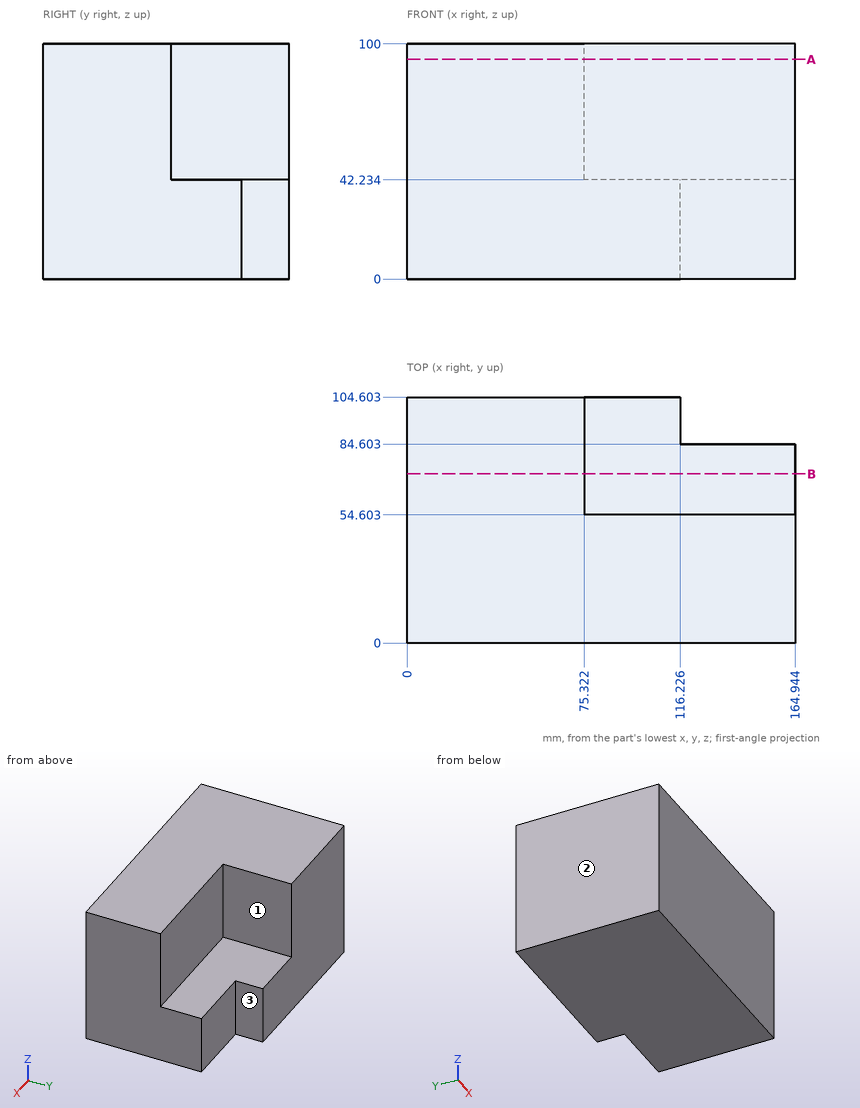
Geometry check sheet. Reference: drawing and pictorial views, mm from the part's lowest x, y, z. A direction names the side the tool comes from. Coordinates: 2 decimals unless noted, no trailing zeros. Order: outer loops, then holes, each group sorted by start corner. A loop starts at its lowest first (then second) coordinate and runs counter-clockwise, first axis right, second up. Notation, with made-up numbers: M 71,49.25 L 109,49.25 A16 cw 109,74.25 Z; hole C 60.25,-37.75 d3. An arc over 180 degrees is marked long. Return JSON: item names as keys, results as strings.
1) Thickness scan on L1, parallel to Z at x = 108, y = 68; L2, parallel to X at y = 94, z = 36; L3, parallel to Y at x = 147, z = 42.5. Record the ranges inside material, lowest first. Write a range as [from, to].
Answer list:
{"L1": "[0, 42.23]", "L2": "[0, 116.23]", "L3": "[0, 54.6]"}
2) Access from +Z, -Z, +X, -X, +Y, -Y to the whole of each face (thin tool, end or side, straight path). Record for the marked faces 1, 2 and 3.
Answer list:
{"face 1": "+Z, +X, +Y", "face 2": "+Z, -Z, -X, +Y, -Y", "face 3": "+Z, -Z, +X, +Y"}
3) Cross-section at A-A, the plane z = 93.5. Record the boundary of the cut face in (x, y), and give its area (3 significant figures).
Answer list:
{"outline": "M 0,0 L 164.94,0 L 164.94,54.6 L 75.32,54.6 L 75.32,104.6 L 0,104.6 Z", "area": "12,800 mm2"}
4) Cross-section at B-B, the plane y = 72. Record the boundary of the cut face in (x, z), and give its area (3 significant figures).
Answer list:
{"outline": "M 0,0 L 164.94,0 L 164.94,42.23 L 75.32,42.23 L 75.32,100 L 0,100 Z", "area": "11,300 mm2"}
5) Gauge pin test, flat ends, axial feed: pin 1 (1 mm diameter, centred on y = 79, z = 50, fed in from +X); pin 2 (2 mm diameter, centred on x = 127, y = 74, fed in from +Z); pin 3 (1.5 mm diameter, centred on x = 95.5, z = 43.5, fed in from +Y). Record the tip position at first contact, or that the pin passes through.
Answer list:
{"pin 1": "x = 75.32", "pin 2": "z = 42.23", "pin 3": "y = 54.6"}
